Answer from the drawing. Dimensions are ordinates in mm from the lowest x, y and z of the part. Give positions to 0.01 mm unless a question says otherwise; leave off trailing zeros. Write each loop counter-clockwise with the first axis right and the second up, starting at its lowest first coordinate (ties: lowest second). Pieces come first, ordered by that corner, then holes. Notation, with made-up numbers: (22, -37) -> (52, -37) arc R17 cw to (52, -9) -> close; hole circle Ø7 at (33, 45.25). An arc over 180 degrees is marked (long way). Put each result on its own line as item: value. Start each with the question number.
1) A flat-ended cylindrical pin translates along its axis: pin 1 Ø1 at (x, y) = (42, 1.5) entering from -Z. Find the tip coordinate at first contact, or state that the pin passes through.
2) A cutting plane is placed at B-B (x = 7.9). Write down the section's boundary in (y, z).
3) A cutting plane is placed at C-C (y = 1.35). Write down the section's boundary in (x, z), then the cut area to 3 significant figures.
4) Find the intervals of material crossed by line 1 along X through (y, z) = (1.75, 4); line 2 along Z through (x, y) = (67.9, 1.3); line 3 along X through (y, z) = (1.85, 5.5), in increasing order. Write a range as from..to.
5) A cutting plane is placed at A-A (z = 4.5). Write down the section's boundary in (x, y), then the cut area to 3 significant figures.
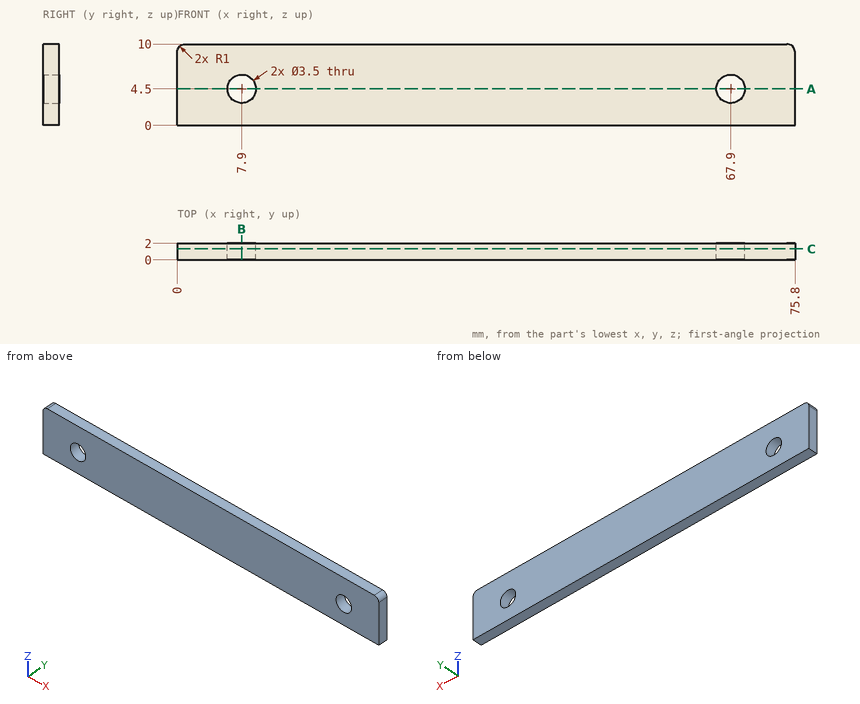
Reply:
1. pin 1: stops at z = 0
2. outline: (0, 0) -> (2, 0) -> (2, 2.75) -> (0, 2.75) -> close; (0, 6.25) -> (2, 6.25) -> (2, 10) -> (0, 10) -> close
3. outline: (0, 0) -> (75.8, 0) -> (75.8, 9) arc R1 ccw to (74.8, 10) -> (1, 10) arc R1 ccw to (0, 9) -> close; hole circle Ø3.5 at (7.9, 4.5); hole circle Ø3.5 at (67.9, 4.5)
3. area: 738 mm2
4. line 1: x = 0..6.22, 9.58..66.22, 69.58..75.8
4. line 2: z = 0..2.75, 6.25..10
4. line 3: x = 0..6.46, 9.34..66.46, 69.34..75.8
5. outline: (0, 0) -> (6.15, 0) -> (6.15, 2) -> (0, 2) -> close; (9.65, 0) -> (66.15, 0) -> (66.15, 2) -> (9.65, 2) -> close; (69.65, 0) -> (75.8, 0) -> (75.8, 2) -> (69.65, 2) -> close
5. area: 138 mm2
